from build123d import *

# Parameters (mm, degrees)
BOSS_EXTRUDE1_DEPTH      = 125
BOSS_EXTRUDE1_DEPTH_BACK = 63.5
SKETCH1_W                = 16
SKETCH1_H                = 16
SKETCH1_W_2              = 14
SKETCH1_H_2              = 14
SKETCH2_R                = 2.1
SKETCH2_R_2              = 1.6
SKETCH2_R_3              = 5.5
CUT_EXTRUDE1_DEPTH       = 127.273512662
CHAMFER1_SIZE            = 1.5


with BuildPart() as part:
    # Sketch1 → Boss-Extrude1 (new, two sides: drawn at the far end of the back side and taken through both)
    with BuildSketch(Plane.XY.offset(-BOSS_EXTRUDE1_DEPTH_BACK)):
        Rectangle(SKETCH1_W, SKETCH1_H)
        Rectangle(SKETCH1_W_2, SKETCH1_H_2, mode=Mode.SUBTRACT)
    extrude(amount=BOSS_EXTRUDE1_DEPTH + BOSS_EXTRUDE1_DEPTH_BACK)

    # Sketch2 → Cut-Extrude1 (cut, through all)
    with BuildSketch(Plane(origin=(0, 8, 0), x_dir=(1, 0, 0), z_dir=(0, 1, 0))):
        with Locations(Location((0, -115.5, 0), (0, 0, 270))):
            Circle(SKETCH2_R)
        with Locations(Location((0, -104.5, 0), (0, 0, 270))):
            Circle(SKETCH2_R_2)
        with Locations(Location((0, 48.5, 0), (0, 0, 270))):
            Circle(SKETCH2_R_3)
        with Locations(Location((0, 60.5, 0), (0, 0, 270))):
            Circle(SKETCH2_R_2)
        with Locations(Location((0, 34.5, 0), (0, 0, 270))):
            Circle(SKETCH2_R_2)
        with Locations(Location((0, -80.5, 0), (0, 0, 270))):
            Circle(SKETCH2_R)
        with Locations(Location((0, -91.5, 0), (0, 0, 270))):
            Circle(SKETCH2_R_2)
    extrude(amount=-CUT_EXTRUDE1_DEPTH, mode=Mode.SUBTRACT)

    # Chamfer1
    # the kernel refuses this chamfer: 1.5 mm, written as the material it takes off along each edge
    with BuildSketch(Plane(origin=(0, 8, 104.5), x_dir=(0, 0, 1), z_dir=(-1, 0, 0))) as chamfer1_piece_1:
        Polygon((1.6 + CHAMFER1_SIZE, 0), (1.6, -CHAMFER1_SIZE), (1.6, 0), align=None)
    revolve(axis=Axis((0, 8, 104.5), (0, 1, 0)), mode=Mode.SUBTRACT)
    with BuildSketch(Plane(origin=(0, 8, 91.5), x_dir=(0, 0, 1), z_dir=(-1, 0, 0))) as chamfer1_piece_2:
        Polygon((1.6 + CHAMFER1_SIZE, 0), (1.6, -CHAMFER1_SIZE), (1.6, 0), align=None)
    revolve(axis=Axis((0, 8, 91.5), (0, 1, 0)), mode=Mode.SUBTRACT)
    with BuildSketch(Plane(origin=(0, -8, 104.5), x_dir=(0, 0, 1), z_dir=(-1, 0, 0))) as chamfer1_piece_3:
        Polygon((1.6 + CHAMFER1_SIZE, 0), (1.6, CHAMFER1_SIZE), (1.6, 0), align=None)
    revolve(axis=Axis((0, -8, 104.5), (0, 1, 0)), mode=Mode.SUBTRACT)
    with BuildSketch(Plane(origin=(0, -8, 91.5), x_dir=(0, 0, 1), z_dir=(-1, 0, 0))) as chamfer1_piece_4:
        Polygon((1.6 + CHAMFER1_SIZE, 0), (1.6, CHAMFER1_SIZE), (1.6, 0), align=None)
    revolve(axis=Axis((0, -8, 91.5), (0, 1, 0)), mode=Mode.SUBTRACT)


solid = part.part
Here's how the part is built. I have some questions about the finished solid (model axes, mm). A direction names the side the tool comes from. Give positions to 0.01 mm unless a question says otherwise; leave off trailing zeros. Order: outer loops, then holes, each group sorted by start corner. A loop starts at its lowest first (then second) coordinate and runs counter-clockwise, first axis right, second up. Notation, with made-up numbers: (3, 65) -> (34, 65) arc R23 cw to (34, 82) -> close; hole circle Ø2 at (49, 28). An arc over 180 degrees is marked (long way). Use a Markdown table: item, result. Add a question column.
Item 1: Imagine slicing it at D-D on z = -60.5. Please give me the cut outline in (x, y).
Item 2: Imagine slicing it at C-C on z = -12.5. Please give me the cut outline in (x, y).
Item 3: Imagine slicing it at A-A on z = 80.5. Please give me the cut outline in (x, y), plus the area to 3 significant figures.
Item 4: If we mould it in two halves opening along X, with no side actions, what happens to faces 1 (the face through (0.07, 7.51, -36.1)), 2 (the face through (0, -8, 29))? For each: pulls with the +X half, pulls with the -X half, needs draft (parallel to the pull), parting line crosses it, or undercut.
Item 5: I need wall thicknesses on line 1 (X direction, y = 6.5, z = 113.5); line 2 (X direction, y = -7.35, z = 80.5). Which ranges of each line are inside material? Lowest first, please.
Item 6: For faces 3 (the face through (0, -7, 29)), 4 (the face through (0, 8, 29)), which set-ups out of +Z, -Z, +X, -X, +Y, -Y let a thin tool reach every point of the face, with its end or its side?
Item 7: Imagine slicing it at B-B on y = 0.5. Please give me the cut outline in (x, z).
Data:
| question | item | result |
|---|---|---|
| 1 | outline | (-8, -8) -> (-1.6, -8) -> (-1.6, -7) -> (-7, -7) -> (-7, 7) -> (-1.6, 7) -> (-1.6, 8) -> (-8, 8) -> close; (1.6, -8) -> (8, -8) -> (8, 8) -> (1.6, 8) -> (1.6, 7) -> (7, 7) -> (7, -7) -> (1.6, -7) -> close |
| 2 | outline | (-8, -8) -> (8, -8) -> (8, 8) -> (-8, 8) -> close; hole (-7, -7) -> (7, -7) -> (7, 7) -> (-7, 7) -> close |
| 3 | outline | (-8, -8) -> (-2.1, -8) -> (-2.1, -7) -> (-7, -7) -> (-7, 7) -> (-2.1, 7) -> (-2.1, 8) -> (-8, 8) -> close; (2.1, -8) -> (8, -8) -> (8, 8) -> (2.1, 8) -> (2.1, 7) -> (7, 7) -> (7, -7) -> (2.1, -7) -> close |
| 3 | area | 51.6 mm² |
| 4 | face 1 | undercut |
| 4 | face 2 | needs draft |
| 5 | line 1 | x = -8 to -7, 7 to 8 |
| 5 | line 2 | x = -8 to -2.1, 2.1 to 8 |
| 6 | face 3 | +Z, -Z |
| 6 | face 4 | +Z, -Z, +X, -X, +Y |
| 7 | outline | (-8, -63.5) -> (-7, -63.5) -> (-7, 125) -> (-8, 125) -> close; (7, -63.5) -> (8, -63.5) -> (8, 125) -> (7, 125) -> close |
